Could you check a few things on this model? Use its own coordinates, in mm. Face numbers are marked on the shaded views. Round coordinates to 2 decimals unless told otherwise and drop trailing zeros. Order: outer loops, then holes, each group sorted by start corner. A loop starts at its lowest first (then second) coordinate and runs counter-clockwise, first axis right, second up. Notation, with made-up numbers: (-11.5, 44.25) - (21.5, 44.25) arc R24 ccw to (21.5, 76.25) - close; hole circle Ø6 at (-7, 35.25). An arc over 180 degrees is marked (long way). Return JSON: item names as keys, results as strings. Group by question number.
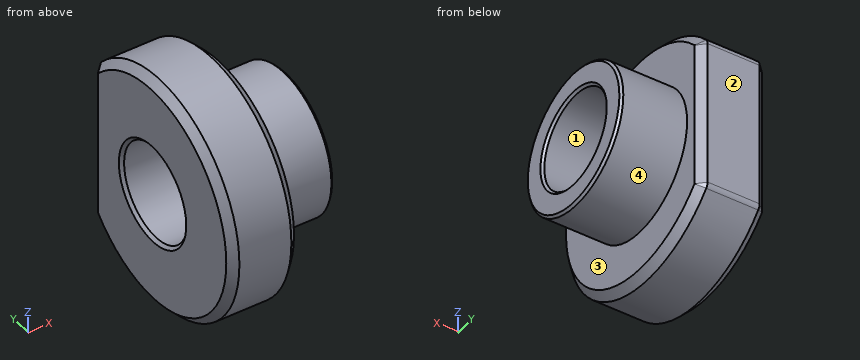
from build123d import *

# Parameters (mm, degrees)
CUT_EXTRUDE_1_REACH = 137.923
CHAMFER_2_SIZE      = 1.5
FILLET_1_R          = 5
CHAMFER_3_SIZE      = 5
CHAMFER_4_SIZE      = 2


with BuildPart() as part:
    # 草图1 → 旋转1 (revolve)
    with BuildSketch(Plane.XY, mode=Mode.PRIVATE) as revolve_1_sk:
        Polygon((0, 30), (0, 75), (43, 75), (43, 45), (85, 45), (85, 30), align=None)
    revolve(revolve_1_sk.sketch.rotate(Axis((0, 0, 0), (1, 0, 0)), 90), axis=Axis((0, 0, 0), (1, 0, 0)))

    # 草图3 → 切除-拉伸1 (cut, up to next)
    with BuildSketch(Plane.ZY, mode=Mode.PRIVATE) as cut_extrude_1_sk1:
        with BuildLine():
            Line((-48.744230428, 57), (48.744230428, 57))
            ThreePointArc((48.744230428, 57), (0, 75), (-48.744230428, 57))
        make_face()
    cut_extrude_1_tool1 = extrude(cut_extrude_1_sk1.sketch, amount=-CUT_EXTRUDE_1_REACH, mode=Mode.PRIVATE) & part.part
    add(cut_extrude_1_tool1.solids().sort_by_distance((0, 64.279608, 0))[0], mode=Mode.SUBTRACT)

    # 倒角2
    chamfer_2_edges = [part.edges().sort_by_distance(p)[0] for p in [
        (85, 0, -30),
        (85, 0, -45),
    ]]
    chamfer(chamfer_2_edges, length=CHAMFER_2_SIZE)

    # 圆角1
    fillet_1_edges = [part.edges().sort_by_distance(p)[0] for p in [
        (21.5, 57, -48.744230428),
        (21.5, 57, 48.744230428),
    ]]
    fillet(fillet_1_edges, radius=FILLET_1_R)

    # 倒角3
    chamfer_3_edges = [part.edges().sort_by_distance(p)[0] for p in [
        (43, -75, 0),
        (0, -75, 0),
        (0, 57, 0),
        (0, 56.667516929, -48.654340969),
        (0, 56.667516929, 48.654340969),
        (43, 57, 0),
        (43, 56.667516929, -48.654340969),
        (43, 56.667516929, 48.654340969),
    ]]
    chamfer(chamfer_3_edges, length=CHAMFER_3_SIZE - 0.0001)  # a hair under: the kernel refuses the full size

    # 倒角4
    chamfer_4_edges = [part.edges().sort_by_distance(p)[0] for p in [
        (0, 0, -30),
    ]]
    chamfer(chamfer_4_edges, length=CHAMFER_4_SIZE)


solid = part.part
1) I want a section at B-B, the plane z = 0. List the corners of the cut face in (x, y) for me, plus the area to 3 significant figures.
2) I want a section at A-A, the plane y = 0. List the corners of the cut face in (x, z) for me, plus the area to 3 significant figures.
3) If I drill on line 1 along Y through (x, z) = (45, 0); line 2 along X through (y, z) = (-34, -44); line 3 along Z through (x, y) = (77.5, -3), over which ranges is the centre line in solid material (lowest first)? Write a range as from..to.
4) I want a section at C-C, the plane x = 78.5. List the corners of the cut face in (y, z) for me.
5) Will these pins go through, and if not, where does the flat tip stop? pin 1 (10 mm diameter, centred on x = 71.5, z = -21.5, fed in from +Y); pin 2 (2 mm diameter, centred on y = -16.5, z = 49, fed in from +X); pin 3 (5 mm diameter, centred on x = 68.5, z = 18.5, fed in from -Y).
6) We'd pull the mould along Y, two halves only. Please class the marked faces 1, 2, 3 and 4: +Y half, -Y half, draft (parallel to the pull), parting line (faces both ways), or undercut.
7) I want a section at D-D, the plane x = 13.5. List the corners of the cut face in (y, z) for me, plus the area to 3 significant figures.
Outcome:
{
 "1": {"outline": "(0, -70) - (5, -75) - (38, -75) - (43, -70) - (43, -45) - (83.5, -45) - (85, -43.5) - (85, -31.5) - (83.5, -30) - (2, -30) - (0, -32) - close; (0, 32) - (2, 30) - (83.5, 30) - (85, 31.5) - (85, 43.5) - (83.5, 45) - (43, 45) - (43, 52) - (38, 57) - (5, 57) - (0, 52) - close", "area": "4,300 mm^2"},
 "2": {"outline": "(0, -70) - (5, -75) - (38, -75) - (43, -70) - (43, -45) - (83.5, -45) - (85, -43.5) - (85, -31.5) - (83.5, -30) - (2, -30) - (0, -32) - close; (0, 32) - (2, 30) - (83.5, 30) - (85, 31.5) - (85, 43.5) - (83.5, 45) - (43, 45) - (43, 70) - (38, 75) - (5, 75) - (0, 70) - close", "area": "5,070 mm^2"},
 "3": {"line 1": "-45..-30, 30..45", "line 2": "0..43", "line 3": "-44.9..-29.85, 29.85..44.9"},
 "4": {"outline": "circle Ø90 at (0, 0); hole circle Ø60 at (0, 0)"},
 "5": {"pin 1": "y = 41.87", "pin 2": "x = 43", "pin 3": "y = -42.06"},
 "6": {"face 1": "undercut", "face 2": "+Y half", "face 3": "draft", "face 4": "parting line"},
 "7": {"outline": "(55.71, -50.21) arc R5 ccw to (57, -46.86) - (57, 46.86) arc R5 ccw to (55.71, 50.21) arc R75 ccw (long way) to start; hole circle Ø60 at (0, 0)", "area": "13,600 mm^2"}
}
